Work out the finished part from the listing and answer in its coordinate system (mm). A direction names the side the tool comes from. Round coordinates to 2 decimals unless told otherwise and drop trailing zeros. Order: outer loops, then holes, each group sorted by start corner. A loop starts at its lowest first (then second) coordinate and runs counter-clockwise, first axis right, second up. Notation, with made-up numbers: (36, 21.25) - (68, 21.25) arc R23 ccw to (68, 54.25) - close; hole circle Ø10 at (-37, 19.5). An arc over 180 degrees is marked (long way). Put each result on its own line as item: value.
```python
from build123d import *

# Parameters (mm, degrees)
SKETCH2_W               = 4.445
SKETCH2_H               = 7.62
PLANETARY_PLATE_R       = 3.25
CUT_EXTRUDE2_DEPTH      = 7.107467815
CUT_EXTRUDE2_DEPTH_BACK = 34.605032185
SKETCH3_R               = 4.3053
CUT_EXTRUDE3_DEPTH      = 8.89
CUT_EXTRUDE4_DEPTH      = 4.445


with BuildPart() as part:
    # Sketch2 → Revolve1 (revolve)
    with BuildSketch(Plane(origin=(0, 0, 0), x_dir=(0, 0, -1), z_dir=(1, 0, 0))):
        with BuildLine():
            Line((18.276532185, 73), (-6.107467815, 73))
            Line((-6.107467815, 73), (-6.107467815, 62.23))
            Line((-6.107467815, 62.23), (11.672532185, 62.23))
            Line((11.672532185, 62.23), (16.117532185, 62.23))
            Line((16.117532185, 62.23), (16.117532185, 54.61))
            Line((16.117532185, 54.61), (16.117532185, 27.016))
            Line((16.117532185, 27.016), (17.133532185, 26))
            Line((17.133532185, 26), (24.605032185, 26))
            Line((24.605032185, 26), (24.605032185, 25))
            Line((24.605032185, 25), (25.605032185, 25))
            Line((25.605032185, 25), (25.605032185, 26))
            Line((25.605032185, 26), (32.589032185, 26))
            Line((32.589032185, 26), (33.605032185, 27.016))
            Line((33.605032185, 27.016), (33.605032185, 31.334))
            Line((33.605032185, 31.334), (32.589032185, 32.35))
            Line((32.589032185, 32.35), (22.467532185, 32.35))
            ThreePointArc((22.467532185, 32.35), (20.222468154, 33.27993597), (19.292532185, 35.525))
            Line((19.292532185, 35.525), (19.292532185, 71.984))
            Line((19.292532185, 71.984), (18.276532185, 73))
        make_face()
        with Locations((13.895032185, 58.42)):
            Rectangle(SKETCH2_W, SKETCH2_H)
    revolve(axis=Axis((0, 0, 0), (0, 0, -1)))

    # Planetary Plate → Cut-Extrude2 (cut, two sides)
    with BuildSketch(Plane.XY) as cut_extrude2_sk:
        with Locations((26.022473401, 62.823808211)):
            Circle(PLANETARY_PLATE_R)
        with Locations((62.823808211, 26.022473401)):
            Circle(PLANETARY_PLATE_R)
        with Locations((62.823808211, -26.022473401)):
            Circle(PLANETARY_PLATE_R)
        with Locations((26.022473401, -62.823808211)):
            Circle(PLANETARY_PLATE_R)
        with Locations((-26.022473401, -62.823808211)):
            Circle(PLANETARY_PLATE_R)
        with Locations((-62.823808211, -26.022473401)):
            Circle(PLANETARY_PLATE_R)
        with Locations((-62.823808211, 26.022473401)):
            Circle(PLANETARY_PLATE_R)
        with Locations((-26.022473401, 62.823808211)):
            Circle(PLANETARY_PLATE_R)
    extrude(amount=CUT_EXTRUDE2_DEPTH, mode=Mode.SUBTRACT)
    extrude(cut_extrude2_sk.sketch, amount=-CUT_EXTRUDE2_DEPTH_BACK, mode=Mode.SUBTRACT)

    # Sketch3 → Cut-Extrude3 (cut)
    with BuildSketch(Plane(origin=(0, 0, -19.292532185), x_dir=(-1, 0, 0), z_dir=(0, 0, -1))):
        with Locations((0, 62.23)):
            Circle(SKETCH3_R)
        with Locations((62.23, 0)):
            Circle(SKETCH3_R)
    extrude(amount=-CUT_EXTRUDE3_DEPTH, mode=Mode.SUBTRACT)

    # Sketch5 → Cut-Extrude4 (cut)
    with BuildSketch(Plane.XY.offset(-11.672532185)):
        with BuildLine():
            ThreePointArc((-6.932957369, 59.067959184), (-8.633427721, 60.862929677), (-11.077660143, 61.236086957))
            ThreePointArc((-11.077660143, 61.236086957), (-44.003254993, 44.003254993), (-61.236086957, 11.077660143))
            ThreePointArc((-61.236086957, 11.077660143), (-60.862929677, 8.633427721), (-59.067959184, 6.932957369))
            ThreePointArc((-59.067959184, 6.932957369), (-55.820664951, 4.121264882), (-54.61, -7.6e-08))
            ThreePointArc((-54.61, -7.6e-08), (-38.615101322, 38.61510132), (7.3e-08, 54.61))
            ThreePointArc((7.3e-08, 54.61), (-4.121264883, 55.820664952), (-6.932957369, 59.067959184))
        make_face()
        with BuildLine():
            ThreePointArc((6.932957369, 59.067959184), (4.121264944, 55.820664991), (7.3e-08, 54.61))
            ThreePointArc((7.3e-08, 54.61), (38.615101322, -38.61510132), (-54.61, -7.6e-08))
            ThreePointArc((-54.61, -7.6e-08), (-55.820664992, -4.121264946), (-59.067959184, -6.932957369))
            ThreePointArc((-59.067959184, -6.932957369), (-60.862929677, -8.633427721), (-61.236086957, -11.077660143))
            ThreePointArc((-61.236086957, -11.077660143), (44.003254993, -44.003254993), (11.077660143, 61.236086957))
            ThreePointArc((11.077660143, 61.236086957), (8.633427721, 60.862929677), (6.932957369, 59.067959184))
        make_face()
    extrude(amount=-CUT_EXTRUDE4_DEPTH, mode=Mode.SUBTRACT)


solid = part.part
```
1) For faces 4 (the flat face through (0.2, 57.6, -11.673)), 5 (the cylindrical face through (0.56, 66.5, -14.91)), 6 (the flat face through (26, -9, -33.605)), determine the directions among +Z, -Z, +X, -X, +Y, -Y from which every point of the face is accessible in a straight line to the end or side of a thin tool.
Findings below:
face 4: +Z
face 5: -Z
face 6: -Z, +X, -X, +Y, -Y
2) A cutting plane is placed at A-A on z = -4. Give the number of separate pieces and of enclosed holes in the cut face, then the cut area to 3 significant figures.
Findings below:
separate pieces: 1
enclosed holes: 9
area: 4,310 mm2
3) For a pull along X with two mould halves and no side action, classify faces 1 (the cylindrical face through (9.717, 30.856, -27.457)), 2 (the flat face through (-54, 32, 6.107)), 3 (the cylindrical face through (8.665, 60.879, -13.864)) as pulls with the +X half, pulls with the -X half, needs draft (parallel to the pull), parting line crosses it, or undercut.
Findings below:
face 1: parting line crosses it
face 2: needs draft
face 3: undercut
4) Straight lines are drawn through the part: L1, parallel to Y at x = -2, z = -1; L2, parallel to X at y = 0, z = 0; L3, parallel to Z at x = 18.5, y = -56.5. For each, find the intervals that lie inside material, in ascending order. Write a range as from..to.
Findings below:
L1: y = -72.97..-62.2, 62.2..72.97
L2: x = -73..-62.23, 62.23..73
L3: z = -19.29..-16.12
5) Given pin 1 Ø6 at (x, y) = (-62.82, -26.02) entering from +Z; pin 2 Ø1.3 at (x, y) = (1, 64.5) entering from -Z; pin 3 Ø2 at (x, y) = (-20, 23.5) entering from +Z; pin 4 Ø8 at (x, z) = (32, -7.5) entering from +Y, each flat-ended and moving along its own axis, determine where each tip first touches the part or whether it passes through.
Findings below:
pin 1: passes through
pin 2: stops at z = -10.4
pin 3: stops at z = -16.12
pin 4: stops at y = 67.42
6) A cutting plane is placed at B-B on z = -30.5. Write down the section's boundary in (x, y).
Findings below:
outline: circle Ø64.7 at (0, 0); hole circle Ø52 at (0, 0)
